Drawing for the job (mm, zero at the part's lowest x, y, z). A direction names the side the tool comes from. Coordinates: 2 decimals unless noted, no trailing zeros. Loops run counter-clockwise (first coordinate to the right, second up) from the corner with the lowest first, then second, coordinate; pieces in that order, holes last. Notation, with made-up numbers: (-29.5, -27) - (4.5, -27) arc R10 ccw to (4.5, -20) - close; hole circle Ø2 at (50.25, 64.25). An arc over 180 degrees is marked (long way). Put each result on its own line as item: value.
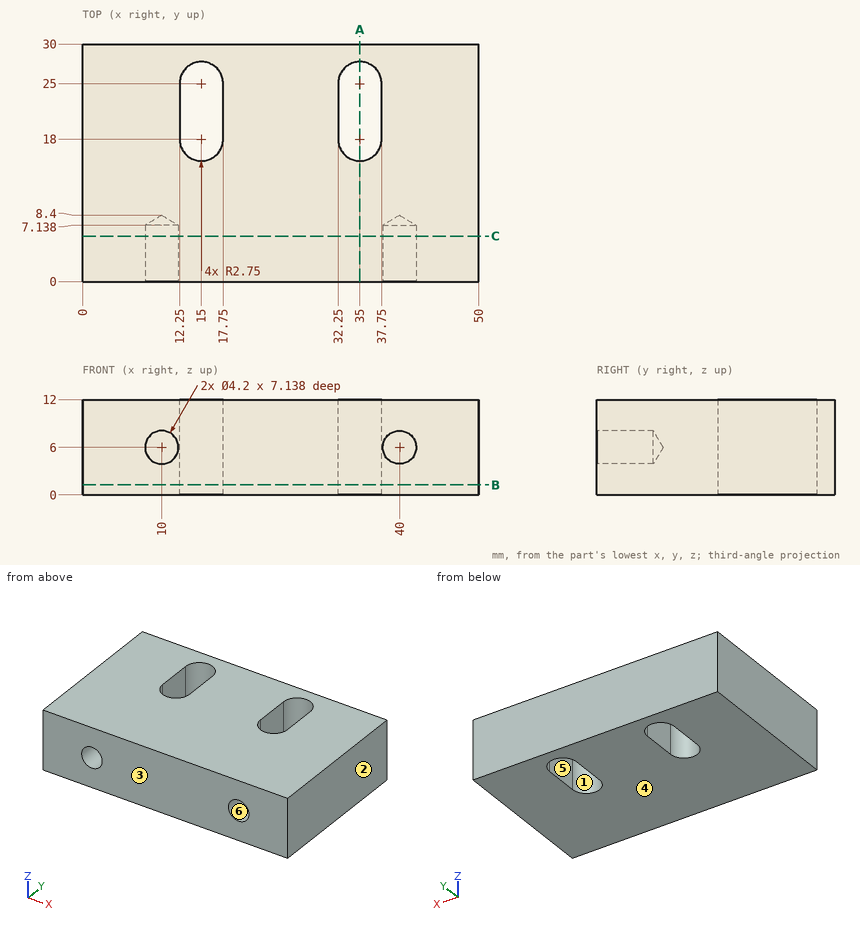
Q1. Slice it at A-A, the plane x = 35. Give the cut face in (y, z), then the cut area to 3 significant figures.
Determined:
outline: (0, 0) - (15.25, 0) - (15.25, 12) - (0, 12) - close; (27.75, 0) - (30, 0) - (30, 12) - (27.75, 12) - close
area: 210 mm2
Q2. Mould opens along X. For the marked faces 1, 2 and 3 say: +X half, -X half, draft (parallel to the pull), parting line (faces both ways), or undercut.
Determined:
face 1: undercut
face 2: +X half
face 3: draft
Q3. Wall check: L1, parallel to X at y = 1.5, z = 6; L2, parallel to X at y = 18, z = 1.25; L3, parallel to Z at x = 40, y = 2.25. Give the ranges that are in metal, low to high. Write a range as from..to.
Determined:
L1: 0..7.9, 12.1..37.9, 42.1..50
L2: 0..12.25, 17.75..32.25, 37.75..50
L3: 0..3.9, 8.1..12
Q4. Slice it at C-C, the plane y = 5.75. Give the cut face in (x, z), then the cut area to 3 significant figures.
Determined:
outline: (0, 0) - (50, 0) - (50, 12) - (0, 12) - close; hole circle Ø4.2 at (10, 6); hole circle Ø4.2 at (40, 6)
area: 572 mm2
Q5. Slice it at B-B, the plane z = 1.25. Give the cut face in (x, y), then the cut area to 3 significant figures.
Determined:
outline: (0, 0) - (50, 0) - (50, 30) - (0, 30) - close; hole (12.25, 18) arc R2.75 ccw to (17.75, 18) - (17.75, 25) arc R2.75 ccw to (12.25, 25) - close; hole (32.25, 18) arc R2.75 ccw to (37.75, 18) - (37.75, 25) arc R2.75 ccw to (32.25, 25) - close
area: 1,380 mm2
Q6. Tool access for the marked faces 4, 5 and 6: list every direction of +Z, -Z, +X, -X, +Y, -Y with a clear straight run to the whole face (end or side of a thin tool).
Determined:
face 4: -Z, +X, -X, +Y, -Y
face 5: +Z, -Z
face 6: -Y
